For this review, take the finished solid that the model builds, in its own axes (mm). A direction names the side the tool comes from. Give positions to 0.01 mm unless a question says otherwise; leave off trailing zeros. Loops run counter-clockwise (first coordinate to the right, second up) from the corner with the lowest first, then second, coordinate; pieces in that order, holes last.
```python
from build123d import *

# Parameters (mm, degrees)
SKETCH_W        = 40
SKETCH_H        = 40
PAD_DEPTH       = 119
SKETCH001_R     = 12.5
PAD001_DEPTH    = 12.5
SKETCH002_W     = 9
SKETCH002_H     = 34
POCKET_DEPTH    = 3
SKETCH003_R     = 1
POCKET001_DEPTH = 8
SKETCH004_W     = 170
SKETCH004_H     = 170
PAD002_DEPTH    = 3


with BuildPart() as part:
    # Sketch → Pad (new body)
    with BuildSketch(Plane.XZ):
        Rectangle(SKETCH_W, SKETCH_H)
    extrude(amount=PAD_DEPTH)

    # Sketch001 (on Face6 of Pad) → Pad001 (join)
    with BuildSketch(Plane.XZ.offset(119)):
        Circle(SKETCH001_R)
    extrude(amount=PAD001_DEPTH)

    # Sketch002 (on Face4 of Pad001) → Pocket (cut)
    with BuildSketch(Plane(origin=(0, 0, 0), x_dir=(1, 0, 0), z_dir=(0, 1, 0))):
        Rectangle(SKETCH002_W, SKETCH002_H)
    extrude(amount=-POCKET_DEPTH, mode=Mode.SUBTRACT)

    # Sketch003 (on Face12 of Pocket) → Pocket001 (cut)
    with BuildSketch(Plane(origin=(0, -3, 0), x_dir=(1, 0, 0), z_dir=(0, 1, 0))):
        with Locations((0, 5.973904)):
            Circle(SKETCH003_R)
        with Locations((0, -6.00258)):
            Circle(SKETCH003_R)
    extrude(amount=-POCKET001_DEPTH, mode=Mode.SUBTRACT)

    # Sketch004 (on Face3 of Pocket001) → Pad002 (join)
    with BuildSketch(Plane(origin=(20, 0, 0), x_dir=(0, 0, 1), z_dir=(1, 0, 0))):
        with Locations((61, 59.5)):
            Rectangle(SKETCH004_W, SKETCH004_H)
    extrude(amount=PAD002_DEPTH)


solid = part.part
```
Q1. Consider section C-C on y = -7.5. Give the boundary of the cut face in (x, z), plus the area to 3 significant figures.
Answers:
outline: (-20, -20) - (20, -20) - (20, -24) - (23, -24) - (23, 146) - (20, 146) - (20, 20) - (-20, 20) - close; hole circle Ø2 at (0, -5.97); hole circle Ø2 at (0, 6)
area: 2,100 mm2
Q2. Machinability: for faces 1 (the flat face through (0, -131.5, 0)), 2 (the flat face through (0, -59, 20)), 3 (the flat face through (0, -59, -20)), which of the approach directions +Z, -Z, +X, -X, +Y, -Y give a long, thin tool a straight path to every point of the face, cutting with its end or side? Answer none if there is none.
Answers:
face 1: +Z, -Z, -X, -Y
face 2: +Z, -X, +Y, -Y
face 3: -Z, -X, +Y, -Y
Q3. For probe 1 along Z at (x, y) = (0, -5.75); probe 2 along Z at (x, y) = (6, -76.5); probe 3 along Y at (x, z) = (-7, -2.5), list the stretches that pass through material, from the lowest coordinate up.
Answers:
probe 1: z = -20 to -6.97, -4.97 to 5, 7 to 20
probe 2: z = -20 to 20
probe 3: y = -131.5 to 0
Q4. Consider section B-B on z = 0. Give the boundary of the cut face in (x, y).
Answers:
outline: (-20, -119) - (-12.5, -119) - (-12.5, -131.5) - (12.5, -131.5) - (12.5, -119) - (20, -119) - (20, -144.5) - (23, -144.5) - (23, 25.5) - (20, 25.5) - (20, 0) - (4.5, 0) - (4.5, -3) - (-4.5, -3) - (-4.5, 0) - (-20, 0) - close
Q5. Consider section A-A on y = -70. Give the boundary of the cut face in (x, z).
Answers:
outline: (-20, -20) - (20, -20) - (20, -24) - (23, -24) - (23, 146) - (20, 146) - (20, 20) - (-20, 20) - close
Q6. Mouldability with a two-part tool opening along X and no side actions: class faces 4 (the flat face through (-5, 0, 0)), 5 (the flat face through (-20, -59, 0)), 6 (the cylindrical face through (11.923, -125.162, 3.755)) as +X half, -X half, draft (parallel to the pull), parting line (faces both ways), or undercut.
Answers:
face 4: draft
face 5: -X half
face 6: undercut
Q7. For pin 1 Ø10 at (x, y) = (8.5, -38.5) entering from +Z; pin 2 Ø2.5 at (x, z) = (0, -5.97) entering from +Y; pin 3 Ø2 at (x, y) = (-4, -17.5) entering from -Z, all flat-tipped, find the tip position at first contact; note any pin that passes through.
Answers:
pin 1: stops at z = 20
pin 2: stops at y = -3
pin 3: stops at z = -20
Q8. Consider section D-D on z = 41.5. Give the boundary of the cut face in (x, y), plus the area to 3 significant figures.
Answers:
outline: (20, -144.5) - (23, -144.5) - (23, 25.5) - (20, 25.5) - close
area: 510 mm2
